The listing builds one solid part. Answer for the finished solid, in the listing's coordinates (mm). Face numbers are marked on the shaded views. A direction names the side the tool comes from. Round coordinates to 2 decimals unless told otherwise and drop trailing zeros. Write each loop counter-clockwise with the first axis right and the second up, starting at its lowest first coordinate (ties: lowest second). Pieces come first, ordered by that corner, then holes. Notation, with made-up numbers: (10, 56.5) - (59, 56.5) arc R10 ccw to (59, 74.5) - close; hole circle Ø3 at (-13.75, 6.5). An arc over 180 degrees is marked (long way). Use a Markdown table: item, result. Add a question column.
1) Each of these flat-tipped pins is pushed along its axis until it touches: P1, Ø6, axis at x = 14.5, y = -17, coming from the +Z side; P2, Ø5.5, axis at x = 6, z = 46.5, coming from the -Y side; P3, Ø14, axis at x = 67.5, y = 8.5, coming from the +Z side (3 decimals). Where does it stop, or does it pass through?
2) A cutting plane is placed at C-C (x = 7). Give the vertices of the cut face in (y, z).
3) A tool of negligible diameter and unlimited length cuts with its end or side. For the marked faces 5, 6, 7 and 8, from which of +Z, -Z, +X, -X, +Y, -Y can it reach the whole face along a straight path? Write none if from no direction.
4) A cutting plane is placed at B-B (z = -8.5). Give the vertices of the cut face in (x, y), then the cut area to 3 significant figures.
5) Find the intervals of material crossed by probe 1 along X at (y, z) = (10.5, 14.5); probe 2 along Z at (x, y) = (46.5, 0), in increasing order. Write a range as from..to.
6) A cutting plane is placed at A-A (y = 0). Give the vertices of the cut face in (x, z) (3 decimals).
7) Determine the mould class of the marked faces 1, 2, 3 and 4 for opening direction X: +X half, -X half, draft (parallel to the pull), parting line (faces both ways), or undercut.
8) A cutting plane is placed at D-D (z = 6.5). Give the vertices of the cut face in (x, y) (3 decimals), then the cut area to 3 significant figures.
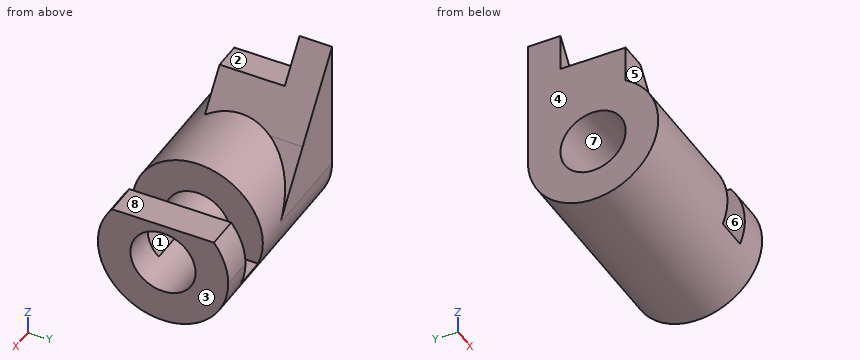
```python
from build123d import *

# Parameters (mm, degrees)
F0_R          = 25.4
F0_R_2        = 12.7
F1_DEPTH      = 76.2
F3_DEPTH      = 25.4
F3_DEPTH_BACK = 12.7
F5_DEPTH      = 25.4
F6_R          = 12.7
F7_DEPTH      = 76.201
F9_DEPTH      = 25.401
F9_DEPTH_BACK = 25.4


with BuildPart() as f1:
    # F0 (on Right) → F1 (new body)
    with BuildSketch(Plane.YZ):
        Circle(F0_R)
        Circle(F0_R_2, mode=Mode.SUBTRACT)
    extrude(amount=F1_DEPTH)

    # F2 (on Front) → F3 (join, two sides)
    with BuildSketch(Plane.XZ) as f3_sk:
        Polygon((0, 22.0133333333), (0, 0), (38.1, 0), (21.59, 22.0133333333), align=None)
        Polygon((0, 50.8), (0, 22.0133333333), (21.59, 22.0133333333), align=None)
    extrude(amount=-F3_DEPTH)
    extrude(f3_sk.sketch, amount=F3_DEPTH_BACK)

    # F4 (on face) → F5 (cut)
    with BuildSketch(Plane.XZ.offset(12.7)):
        Polygon((0, 50.8), (0, 36.3985226281), (10.801108029, 36.3985226281), align=None)
    extrude(amount=-F5_DEPTH, mode=Mode.SUBTRACT)

    # F6 (on Right) → F7 (cut, through all)
    with BuildSketch(Plane.YZ):
        Circle(F6_R)
    extrude(amount=F7_DEPTH, mode=Mode.SUBTRACT)

    # F8 (on Front) → F9 (cut, two sides)
    with BuildSketch(Plane.XZ) as f9_sk:
        Polygon((76.2, 25.4), (50.8, 25.4), (50.8, -9.525), (63.5, -9.525), (63.5, 15.875), (76.2, 15.875), align=None)
    extrude(amount=-F9_DEPTH, mode=Mode.SUBTRACT)
    extrude(f9_sk.sketch, amount=F9_DEPTH_BACK, mode=Mode.SUBTRACT)


solid = f1.part
```
Entries:
| question | item | result |
|---|---|---|
| 1 | P1 | stops at z = 21.19 |
| 1 | P2 | stops at y = 12.7 |
| 1 | P3 | stops at z = 15.875 |
| 2 | outline | (-12.7, 22) arc R25.4 ccw (long way) to (25.4, 0) - (25.4, 41.47) - (12.7, 41.47) - (12.7, 36.4) - (-12.7, 36.4) - close; hole circle Ø25.4 at (0, 0) |
| 3 | face 5 | +Z, +X, -X, -Y |
| 3 | face 6 | +Z, +Y, -Y |
| 3 | face 7 | +X, -X |
| 3 | face 8 | +Z, +X, +Y, -Y |
| 4 | outline | (0, -23.94) - (50.8, -23.94) - (50.8, -9.44) - (0, -9.44) - close; (0, 9.44) - (50.8, 9.44) - (50.8, 23.94) - (0, 23.94) - close; (63.5, -23.94) - (76.2, -23.94) - (76.2, -9.44) - (63.5, -9.44) - close; (63.5, 9.44) - (76.2, 9.44) - (76.2, 23.94) - (63.5, 23.94) - close |
| 4 | area | 1,840 mm² |
| 5 | probe 1 | x = 0..50.8, 63.5..76.2 |
| 5 | probe 2 | z = -25.4..-12.7, 12.7..25.4 |
| 6 | outline | (0, -25.4) - (76.2, -25.4) - (76.2, -12.7) - (0, -12.7) - close; (0, 12.7) - (50.8, 12.7) - (50.8, 25.4) - (19.05, 25.4) - (10.801, 36.399) - (0, 36.399) - close; (63.5, 12.7) - (76.2, 12.7) - (76.2, 15.875) - (63.5, 15.875) - close |
| 7 | face 1 | undercut |
| 7 | face 2 | draft |
| 7 | face 3 | +X half |
| 7 | face 4 | -X half |
| 8 | outline | (0, -24.554) - (50.8, -24.554) - (50.8, -10.911) - (0, -10.911) - close; (0, 10.911) - (50.8, 10.911) - (50.8, 24.554) - (33.225, 24.554) - (33.225, 25.4) - (0, 25.4) - close; (63.5, -24.554) - (76.2, -24.554) - (76.2, -10.911) - (63.5, -10.911) - close; (63.5, 10.911) - (76.2, 10.911) - (76.2, 24.554) - (63.5, 24.554) - close |
| 8 | area | 1,760 mm² |
